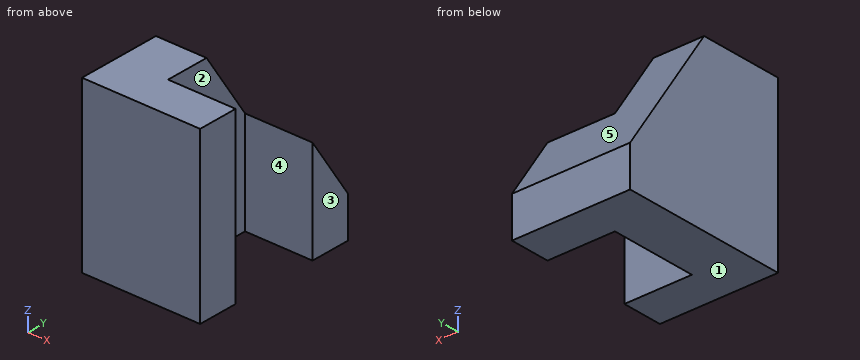
Autodesk Fusion 360 part; units mm, degrees
sketch "Sketch1" plane through (0, 0, 0) normal (0, 0, 1) x (1, 0, 0)
  line L0 (0, 0) -> (0, 25)
  line L1 (0, 25) -> (15, 25)
  line L2 (15, 25) -> (15, 12)
  line L3 (15, 12) -> (35, 12)
  line L4 (35, 12) -> (35, 0)
  line L5 (35, 0) -> (0, 0)
  dimension "d1" = 25
  dimension "d2" = 20
  dimension "d3" = 35
  dimension "d4" = 12
extrude "Extrude1" add sketch "Sketch1" along normal mid plane 50
sketch "Sketch2" plane through (0, 0, 0) normal (-1, 0, 0) x (0, 0, 1)
  line L0 (-25, 0) -> (25, 0)
  line L1 (25, 0) -> (25, 25)
  line L2 (25, 25) -> (-25, 25)
  line L3 (-25, 25) -> (-25, 0)
  line L4 (-25, 25) -> (-25, 50)
  line L5 (-25, 50) -> (-13, 50)
  line L6 (-13, 50) -> (25, 25)
  dimension "d7" = 25
  dimension "d8" = 12
extrude "Extrude2" add sketch "Sketch2" against normal blind 15 contours L2 L4 L5 L6
sketch "Sketch3" plane through (15, 0, 0) normal (1, 0, 0) x (0, 0, -1)
  line L0 (-25, 25) -> (-25, 12)
  line L1 (-25, 12) -> (25, 12)
  line L2 (25, 12) -> (25, 50)
  line L3 (25, 50) -> (13, 50)
  line L4 (13, 50) -> (-25, 25)
  line L5 (-5.24, 38) -> (25, 38)
  dimension "d11" = 12
extrude "Extrude3" add sketch "Sketch3" along normal blind 20 contours L2 L3 L4 L5
Work out the finished part from the listing and answer in its coordinate system (mm). Face numbers are marked on the shaded views. A direction names the side the tool comes from. Give positions to 0.01 mm unless a question says otherwise; leave off trailing zeros. Loops run counter-clockwise (first coordinate to the right, second up) from the corner with the lowest first, then second, coordinate; pieces in that order, holes last. Notation, with made-up numbers: (73.5, 84) - (101.5, 84) arc R8 cw to (101.5, 92) - close; hole circle Ø5 at (49, 72). An arc over 180 degrees is marked (long way). Answer in a Markdown table with one row per item. Add a question column.
Q1. The part is cut by section A-A (x = 31). Determine the outline of the cut face in (y, z).
Q2. A tool of negligible diameter and unlimited length cuts with its end or side. For the marked faces 1 and 2, from which of +Z, -Z, +X, -X, +Y, -Y can it reach the whole face along a straight path? Write none if from no direction.
Q3. The part is cut by section D-D (x = 7). Determine the outline of the cut face in (y, z).
Q4. Consider line 1 along X through (y, z) = (28, -3); line 2 along Z through (x, y) = (10, 30.5); line 3 along Y through (x, z) = (25.5, 19.5). Determine where each line is inside the solid, lowest interval first.
Q5. Determine the mould class of the marked faces 3, 4 and 5 for opening direction Y: released by +Y, released by -Y, zero draft, split by the parting line, or undercut.
Q6. The part is cut by section C-C (y = 47). Determine the outline of the cut face in (x, z).
Q7. Each of these flat-tipped pins is pushed along its axis until it touches: P1, Ø2, axis at x = 22.5, y = 39.5, coming from the +Z side; P2, Ø5, axis at x = 18.5, y = 29.5, coming from the -Z side; P3, Ø5, axis at x = 23, z = 16.5, coming from the +Y side. Where does it stop, or does it pass through?
Q8. The part is cut by section B-B (z = -15.5). Determine the outline of the cut face in (x, y), and give its area (3 significant figures).
Solution:
| question | item | result |
|---|---|---|
| 1 | outline | (0, -25) - (12, -25) - (12, 25) - (0, 25) - close; (38, -25) - (50, -25) - (50, -13) - (38, 5.24) - close |
| 2 | face 1 | -Z, +X, -X, +Y, -Y |
| 2 | face 2 | +Z, -Z, +X |
| 3 | outline | (0, -25) - (50, -25) - (50, -13) - (25, 25) - (0, 25) - close |
| 4 | line 1 | x = 0 to 15 |
| 4 | line 2 | z = -25 to 16.64 |
| 4 | line 3 | y = 0 to 12 |
| 5 | face 3 | zero draft |
| 5 | face 4 | undercut |
| 5 | face 5 | released by +Y |
| 6 | outline | (0, -25) - (35, -25) - (35, -8.44) - (0, -8.44) - close |
| 7 | P1 | stops at z = 4.48 |
| 7 | P2 | passes through |
| 7 | P3 | stops at y = 12 |
| 8 | outline | (0, 0) - (35, 0) - (35, 12) - (15, 12) - (15, 38) - (35, 38) - (35, 50) - (0, 50) - close |
| 8 | area | 1,230 mm² |
